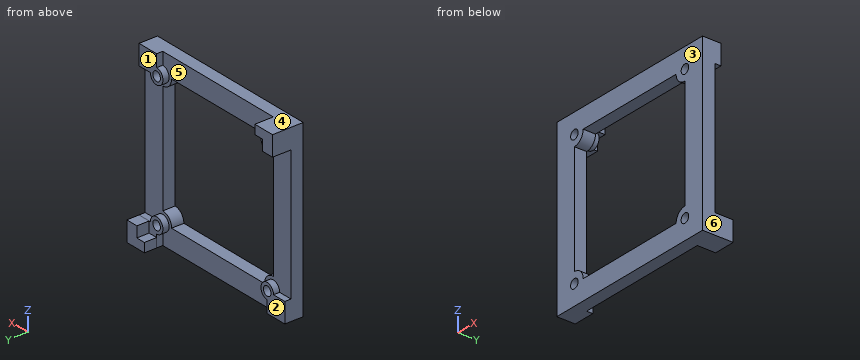
from build123d import *

# Parameters (mm, degrees)
EXTRUDE_1_DEPTH      = 3
EXTRUDE_1_DEPTH_BACK = 53
SKETCH_1_W           = 58
SKETCH_1_H           = 4
SKETCH_2_R           = 1.5
CUT_EXTRUDE_1_DEPTH  = 53
EXTRUDE_START        = 2
SKETCH_3_R           = 2.5
SKETCH_3_R_2         = 1.5
EXTRUDE_2_DEPTH      = 2
CUT_EXTRUDE_2_DEPTH  = 9
EXTRUDE_3_DEPTH      = 2
EXTRUDE_4_DEPTH      = 4


with BuildPart() as part:
    # 草图1 → 凸台-拉伸1 (new, two sides: drawn at the far end of the back side and taken through both)
    with BuildSketch(Plane.XY.offset(-EXTRUDE_1_DEPTH_BACK)):
        with Locations((0, -2)):
            Rectangle(SKETCH_1_W, SKETCH_1_H)
    extrude(amount=EXTRUDE_1_DEPTH + EXTRUDE_1_DEPTH_BACK)

    # 草图2 → 切除-拉伸1 (cut)
    with BuildSketch(Plane(origin=(0, 0, 0), x_dir=(1, 0, 0), z_dir=(0, 1, 0))):
        with Locations(Location((-22, 46.5, 0), (0, 0, 180))):
            Circle(SKETCH_2_R)
        with Locations(Location((22, 46.5, 0), (0, 0, 180))):
            Circle(SKETCH_2_R)
        with Locations(Location((22, 3.5, 0), (0, 0, 180))):
            Circle(SKETCH_2_R)
        with Locations(Location((-22, 3.5, 0), (0, 0, 180))):
            Circle(SKETCH_2_R)
    extrude(amount=-CUT_EXTRUDE_1_DEPTH, mode=Mode.SUBTRACT)

    # 草图3 → 凸台-拉伸2 (add)
    # profile 1 of 4: a face of its own
    with BuildSketch(Plane(origin=(0, 0, 0), x_dir=(1, 0, 0), z_dir=(0, 1, 0)).offset(EXTRUDE_START)):
        with Locations((-22, 46.5)):
            Circle(SKETCH_3_R)
        with Locations(Location((-22, 46.5, 0), (0, 0, 180))):
            Circle(SKETCH_3_R_2, mode=Mode.SUBTRACT)
    # profile 2 of 4: a face of its own
    with BuildSketch(Plane(origin=(0, 0, 0), x_dir=(1, 0, 0), z_dir=(0, 1, 0)).offset(EXTRUDE_START)):
        with Locations((22, 46.5)):
            Circle(SKETCH_3_R)
        with Locations(Location((22, 46.5, 0), (0, 0, 180))):
            Circle(SKETCH_3_R_2, mode=Mode.SUBTRACT)
    # profile 3 of 4: a face of its own
    with BuildSketch(Plane(origin=(0, 0, 0), x_dir=(1, 0, 0), z_dir=(0, 1, 0)).offset(EXTRUDE_START)):
        with Locations((22, 3.5)):
            Circle(SKETCH_3_R)
        with Locations(Location((22, 3.5, 0), (0, 0, 180))):
            Circle(SKETCH_3_R_2, mode=Mode.SUBTRACT)
    # profile 4 of 4: a face of its own
    with BuildSketch(Plane(origin=(0, 0, 0), x_dir=(1, 0, 0), z_dir=(0, 1, 0)).offset(EXTRUDE_START)):
        with Locations((-22, 3.5)):
            Circle(SKETCH_3_R)
        with Locations(Location((-22, 3.5, 0), (0, 0, 180))):
            Circle(SKETCH_3_R_2, mode=Mode.SUBTRACT)
    extrude(amount=-EXTRUDE_2_DEPTH)

    # 草图4 → 切除-拉伸2 (cut)
    with BuildSketch(Plane(origin=(0, 0, 0), x_dir=(1, 0, 0), z_dir=(0, 1, 0))):
        with BuildLine():
            Line((-18.5, 46.56), (18.5, 46.5))
            ThreePointArc((18.5, 46.5), (19.525126266, 44.025126266), (22, 43))
            Line((22, 43), (22, 7))
            ThreePointArc((22, 7), (19.525126266, 5.974873734), (18.5, 3.5))
            Line((18.5, 3.5), (-18.5, 3.44))
            ThreePointArc((-18.5, 3.44), (-19.503639564, 5.953932471), (-22, 7.000514248))
            Line((-22, 7.000514248), (-22, 42.999485752))
            ThreePointArc((-22, 42.999485752), (-19.503639564, 44.046067529), (-18.5, 46.56))
        make_face()
    extrude(amount=-CUT_EXTRUDE_2_DEPTH, mode=Mode.SUBTRACT)

    # 草图5 → 凸台-拉伸3 (add)
    with BuildSketch(Plane(origin=(0, 0, 0), x_dir=(1, 0, 0), z_dir=(0, 1, 0))):
        Polygon((-22, 49), (-22, 53), (-29, 53), (-29, 46.5), (-24.5, 46.5), align=None)
        Polygon((22, 49), (22, 53), (29, 53), (29, 46.5), (24.5, 46.5), align=None)
        Polygon((24.5, 3.5), (29, 3.5), (29, -3), (22, -3), (22, 1), align=None)
        Polygon((-24.5, 3.5), (-29, 3.5), (-29, -3), (-22, -3), (-22, 1), align=None)
    extrude(amount=EXTRUDE_3_DEPTH)

    # 草图6 → 凸台-拉伸4 (add)
    with BuildSketch(Plane(origin=(0, 2, 0), x_dir=(1, 0, 0), z_dir=(0, 1, 0))):
        Polygon((-24.979953432, 3.5), (-24.979953432, 0), (-22, 0), (-22, -3), (-29, -3), (-29, 3.5), align=None)
        Polygon((21.985616423, 50), (25, 50), (25, 46.500843785), (29, 46.5), (29, 53), (22, 53), align=None)
    extrude(amount=EXTRUDE_4_DEPTH)


solid = part.part
For this review, take the finished solid that the model builds, in its own axes (mm). Face numbers are marked on the shaded views. A direction names the side the tool comes from. Give positions to 0.01 mm unless a question says otherwise; leave off trailing zeros. Loops run counter-clockwise (first coordinate to the right, second up) from the corner with the lowest first, then second, coordinate; pieces in that order, holes last. Notation, with made-up numbers: M 88.25,16 L 115.25,16 A11 cw 115.25,31 Z; hole C 1.5,10.25 d5. An arc over 180 degrees is marked long. Answer as a JSON object with one key per item and string values. Group by question number.
Q1. For probe 1 along X at (y, z) = (-3.5, -35.5); probe 2 along Y at (x, z) = (-25.5, -40.5); probe 3 along X at (y, z) = (-1, -47.5), list the stretches that pass through material, from the lowest coordinate up. Write a range as [from, to].
Q2. Add section B-B on z = -21. Give the boundary of the cut face in (x, y).
Q3. Insertion check: P1, Ø5, axis at x = -28, y = 4, coming from the -Z side; P2, Ø5, axis at x = -22, z = -3.5, coming from the +Y side; P3, Ø4, axis at y = 4.5, z = -2.5, coming from the +X side. Each pin has a flat end and moves straight along its axis. Give the tip position at first contact, or say it passes through.
Q4. Add section A-A on y = -1.5. Give the boundary of the cut face in (x, z), and give its area (3 significant figures).
Q5. Mouldability with a two-part tool opening along X and no side actions: class the marked faces 4, 5 and 6 as +X half, -X half, draft (parallel to the pull), parting line (faces both ways), or undercut.
Q6. Tool access review of the marked faces 1, 2 and 3: name each direction out of +Z, -Z, +X, -X, +Y, -Y from which nothing blocks a thin tool from reaching the whole face with its end or side.
Q7. Add section C-C on x = 9.5. Give the boundary of the cut face in (y, z), and give its area (3 significant figures).
Checked values:
{
 "1": {"probe 1": "[-29, -22], [22, 29]", "probe 2": "[-4, 0]", "probe 3": "[-29, -23.12], [-20.88, 20.88], [23.12, 29]"},
 "2": {"outline": "M -29,-4 L -22,-4 L -22,0 L -29,0 Z; M 22,-4 L 29,-4 L 29,0 L 22,0 Z"},
 "3": {"P1": "z = -53", "P2": "y = 2", "P3": "x = -24.98"},
 "4": {"outline": "M -29,-53 L 29,-53 L 29,3 L -29,3 Z; hole C -22,-46.5 d3; hole C -22,-3.5 d3; hole M -22,-43 A3.5 cw -18.5,-46.56 L 18.5,-46.5 A3.5 cw 22,-43 L 22,-7 A3.5 cw 18.5,-3.5 L -18.5,-3.44 A3.5 cw -22,-7 Z; hole C 22,-46.5 d3; hole C 22,-3.5 d3", "area": "1,360 mm²"},
 "5": {"face 4": "draft", "face 5": "undercut", "face 6": "+X half"},
 "6": {"face 1": "+Z, +X, +Y", "face 2": "-Z, -X, +Y", "face 3": "+Z, -Z, +X, -X, -Y"},
 "7": {"outline": "M -4,-53 L 0,-53 L 0,-46.51 L -4,-46.51 Z; M -4,-3.49 L 0,-3.49 L 0,3 L -4,3 Z", "area": "51.9 mm²"}
}
